Could you check a few things on this model? Use its own coordinates, in mm. Face numbers are marked on the shaded views. A direction names the side the tool comes from. Round coordinates to 2 decimals unless told otherwise and drop trailing zeros. Order: outer loops, then holes, each group sorted by start corner. A loop starts at its lowest first (then second) coordinate and runs counter-clockwise, first axis right, second up.
```python
from build123d import *

# Parameters (mm, degrees)
EXTRUDE_THIN1_START     = -6.35
EXTRUDE_THIN1_DEPTH     = 12.7
SKETCH4_R               = 2.2479
EXTRUDE3_DEPTH          = 29.141606724
SKETCH6_R               = 2.2479
CUT_EXTRUDE1_DEPTH      = 31.618591166
CUT_EXTRUDE2_DEPTH      = 29.141606724
CUT_EXTRUDE2_DEPTH_BACK = 29.141606724
CUT_EXTRUDE3_DEPTH      = 31.618591166
CUT_EXTRUDE3_DEPTH_BACK = 31.618591166


# Read off the part's stored shape, not the designer's step: Extrude-Thin1
with BuildPart() as part:
    # Extrude-Thin1 outline → Extrude-Thin1 (new body)
    with BuildSketch(Plane(origin=(0, 0, 0), x_dir=(1, 0, 0), z_dir=(0, 1, 0)).offset(EXTRUDE_THIN1_START)):
        with BuildLine():
            Line((4.572, -3.048), (25.4, -3.048))
            Line((25.4, -3.048), (25.4, 0))
            Line((25.4, 0), (4.572, 0))
            ThreePointArc((4.572, 0), (1.339107796, -1.339107796), (0, -4.572))
            Line((0, -4.572), (0, -15.875))
            Line((0, -15.875), (3.048, -15.875))
            Line((3.048, -15.875), (3.048, -4.572))
            ThreePointArc((3.048, -4.572), (3.494369265, -3.494369265), (4.572, -3.048))
        make_face()
    extrude(amount=EXTRUDE_THIN1_DEPTH)

    # Sketch4 → Extrude3 (cut, through all)
    with BuildSketch(Plane(origin=(3.048, 0, 0), x_dir=(0, 0, -1), z_dir=(1, 0, 0))):
        with Locations((-7.975, 0)):
            Circle(SKETCH4_R)
    extrude(amount=-EXTRUDE3_DEPTH, mode=Mode.SUBTRACT)

    # Sketch6 → Cut-Extrude1 (cut, through all)
    with BuildSketch(Plane.XY):
        with Locations(Location((16.4, 0, 0), (0, 0, 180))):
            Circle(SKETCH6_R)
    extrude(amount=CUT_EXTRUDE1_DEPTH, mode=Mode.SUBTRACT)

    # Sketch8 → Cut-Extrude2 (cut, two sides: drawn at the far end of the back side and taken through both)
    with BuildSketch(Plane(origin=(3.048, 0, 0), x_dir=(0, 0, -1), z_dir=(1, 0, 0)).offset(-CUT_EXTRUDE2_DEPTH_BACK)):
        with BuildLine():
            Line((12.319806212, 46.222872755), (-13.97, 6.35))
            ThreePointArc((-13.97, 6.35), (-15.875, 0), (-13.97, -6.35))
            Line((-13.97, -6.35), (12.319806212, -46.222872755))
            Line((12.319806212, -46.222872755), (-83.199823025, -46.222872755))
            Line((-83.199823025, -46.222872755), (-83.199823025, 46.222872755))
            Line((-83.199823025, 46.222872755), (12.319806212, 46.222872755))
        make_face()
    extrude(amount=CUT_EXTRUDE2_DEPTH + CUT_EXTRUDE2_DEPTH_BACK, mode=Mode.SUBTRACT)

    # Sketch9 → Cut-Extrude3 (cut, two sides: drawn at the far end of the back side and taken through both)
    with BuildSketch(Plane.XY.offset(-CUT_EXTRUDE3_DEPTH_BACK)):
        with BuildLine():
            Line((-11.412637658, 59.293250448), (23.495, 6.35))
            ThreePointArc((23.495, 6.35), (25.4, 0), (23.495, -6.35))
            Line((23.495, -6.35), (-11.412637658, -59.293250448))
            Line((-11.412637658, -59.293250448), (115.418445833, -59.293250448))
            Line((115.418445833, -59.293250448), (115.418445833, 59.293250448))
            Line((115.418445833, 59.293250448), (-11.412637658, 59.293250448))
        make_face()
    extrude(amount=CUT_EXTRUDE3_DEPTH + CUT_EXTRUDE3_DEPTH_BACK, mode=Mode.SUBTRACT)


solid = part.part
```
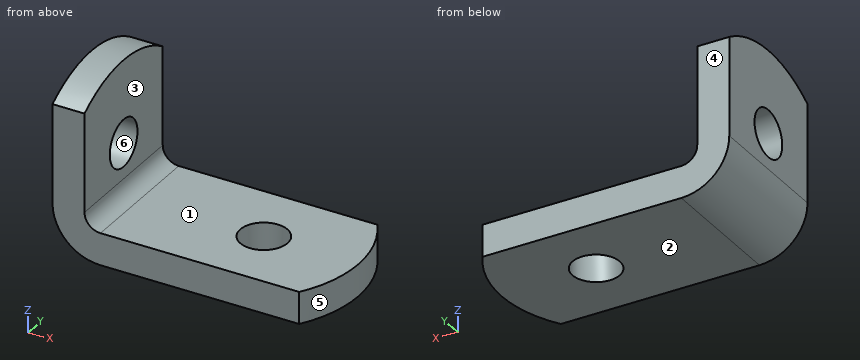
Q1. Imagine slicing it at C-C, the plane z = 6.25. Please give me the cut outline in (x, y), then the cut area to 3 significant figures.
Q2. I need wall thicknesses on L1, parallel to Y at x = 16.4, z = 1.4; L2, parallel to X at y = -4, z = 5.5. Which ranges of each line are inside material? Lowest first, please.
Q3. For P1, Ø5.5, axis at y = 0, z = 9.5, coming from the +X side, with a flat end and sliding along its axis, tell me the tip position at first contact or that it passes through.
Q4. We'd pull the mould along Y, two halves only. Please class the marked faces 3, 4, 5 and 6: released by +Y, released by -Y, zero draft, split by the parting line, or undercut.
Q5. Imagine slicing it at A-A, the plane x = 16.4. Please give me the cut outline in (y, z), then the cut area to 3 significant figures.
Q6. Imagine slicing it at D-D, the plane y = 4.5. Please give me the cut outline in (x, z), then the cut area to 3 significant figures.
Q7. Imagine slicing it at B-B, the plane y = 0. Please give me the cut outline in (x, z) (3 decimals), then the cut area to 3 significant figures.
Q8. For the marked faces 1 and 2, which set-ups out of +Z, -Z, +X, -X, +Y, -Y let a thin tool reach every point of the face, with its end or its side?
Filled in:
1. outline: (0, -6.35) - (3.05, -6.35) - (3.05, -1.44) - (0, -1.44) - close; (0, 1.44) - (3.05, 1.44) - (3.05, 6.35) - (0, 6.35) - close
1. area: 29.9 mm2
2. L1: y = -6.35 to -2.25, 2.25 to 6.35
2. L2: x = 0 to 3.05
3. P1: stops at x = 3.05
4. face 3: zero draft
4. face 4: released by +Y
4. face 5: split by the parting line
4. face 6: undercut
5. outline: (-6.35, 0) - (-2.25, 0) - (-2.25, 3.05) - (-6.35, 3.05) - close; (2.25, 0) - (6.35, 0) - (6.35, 3.05) - (2.25, 3.05) - close
5. area: 25.0 mm2
6. outline: (0, 4.57) arc R4.57 ccw to (4.57, 0) - (24.49, 0) - (24.49, 3.05) - (4.57, 3.05) arc R1.52 cw to (3.05, 4.57) - (3.05, 14.96) - (0, 14.96) - close
6. area: 107 mm2
7. outline: (0, 4.572) arc R4.572 ccw to (4.572, 0) - (14.152, 0) - (14.152, 3.048) - (4.572, 3.048) arc R1.524 cw to (3.048, 4.572) - (3.048, 5.727) - (0, 5.727) - close; (0, 10.223) - (3.048, 10.223) - (3.048, 15.875) - (0, 15.875) - close; (18.648, 0) - (25.4, 0) - (25.4, 3.048) - (18.648, 3.048) - close
7. area: 85.1 mm2
8. face 1: +Z, +X, +Y, -Y
8. face 2: -Z, +X, -X, +Y, -Y
